Read the model definition and answer for the solid it produces. Units are mm, in the model's axes. Face numbers are marked on the shaded views. Coordinates: 2 decimals unless noted, no trailing zeros. Order: outer loops, then holes, each group sorted by start corner. A loop starts at its lowest first (then second) coordinate and runs counter-clockwise, first axis right, second up. Notation, with made-up numbers: M 82,-38.5 L 100,-38.5 A29 ccw 100,-3.5 Z; hole C -16,-15.75 d11. An arc over 180 degrees is marked long. One line per question, with ' | ' between items. Start each with the question number.
1) The mould has two halves that part along X. Classify the marked faces 1, 2, 3 and 4: +X half, -X half, draft (parallel to the pull), parting line (faces both ways), or undercut.
2) Find section C-C, the plane z = 15.5. Write down the section's boundary in (x, y), plus the area to 3 significant figures.
3) Find section A-A, the plane x = 10.6. Write down the section's boundary in (y, z).
4) Given P1, Ø3, axis at x = -1, z = 12, coming from the -Y side; P2, Ø1.5, axis at y = 19, z = 2, coming from the -X side; P3, Ø2, axis at x = 24.5, y = -23.5, coming from the +Z side, each flat-ended and moving along its own axis, determine where each tip first touches the part or whether it passes through.
5) Find section D-D, the plane x = 0. Write down the section's boundary in (y, z), plus the area to 3 significant figures.
6) Consider probe 1 along Y at (x, z) = (0, 10.25); probe 2 along Y at (x, z) = (0, 1.5); probe 3 along Z at (x, y) = (14, -30). Determine where each line is inside the solid, lowest interval first.
7) Find section B-B, the plane y = -16. Write down the section's boundary in (x, z), plus the area to 3 significant figures.
from build123d import *

# Parameters (mm, degrees)
ESQUISSE1_R             = 35
BOSS_EXTRU_1_DEPTH      = 5
ENL_V_MAT_EXTRU_1_REACH = 51.749
BOSS_EXTRU_3_OUTLINE_R  = 4.75
BOSS_EXTRU_3_DEPTH      = 12


# Read off the part's stored shape, not the designer's step: Boss.-Extru.3
with BuildPart() as part:
    # Esquisse1 → Boss.-Extru.1 (new body)
    with BuildSketch(Plane.XY):
        Circle(ESQUISSE1_R)
        with BuildLine():
            ThreePointArc((4.728110875, -10.282810642), (4.727635283, -10.351772147), (4.726208599, -10.420720532))
            Line((4.726208599, -10.420720532), (4.312478928, -25.415013705))
            ThreePointArc((4.312478928, -25.415013705), (-0.823528687, -30.275201539), (-5.683716521, -25.139193925))
            Line((-5.683716521, -25.139193925), (-5.26998685, -10.144900751))
            ThreePointArc((-5.26998685, -10.144900751), (-0.202927621, -5.283286233), (4.728110875, -10.282810642))
        make_face(mode=Mode.SUBTRACT)
        with BuildLine():
            Line((-8.268845484, -10.062154817), (-8.682575156, -25.05644799))
            ThreePointArc((-8.682575156, -25.05644799), (-11.353299115, -27.583745664), (-13.880596789, -24.913021704))
            Line((-13.880596789, -24.913021704), (-13.466867118, -9.918728531))
            ThreePointArc((-13.466867118, -9.918728531), (-10.796143158, -7.391430858), (-8.268845484, -10.062154817))
        make_face(mode=Mode.SUBTRACT)
        with BuildLine():
            Line((12.923088867, -10.646892753), (12.509359196, -25.641185926))
            ThreePointArc((12.509359196, -25.641185926), (9.838635236, -28.168483599), (7.311337562, -25.49775964))
            Line((7.311337562, -25.49775964), (7.725067233, -10.503466467))
            ThreePointArc((7.725067233, -10.503466467), (10.395791193, -7.976168793), (12.923088867, -10.646892753))
        make_face(mode=Mode.SUBTRACT)
        with BuildLine():
            Line((-13.2, 10), (-13.2, 25))
            ThreePointArc((-13.2, 25), (-10.6, 27.6), (-8, 25))
            Line((-8, 25), (-8, 10))
            ThreePointArc((-8, 10), (-10.6, 7.4), (-13.2, 10))
        make_face(mode=Mode.SUBTRACT)
        with BuildLine():
            ThreePointArc((5, 10), (0, 5), (-5, 10))
            Line((-5, 10), (-5, 25))
            ThreePointArc((-5, 25), (0, 30), (5, 25))
            Line((5, 25), (5, 10))
        make_face(mode=Mode.SUBTRACT)
        with BuildLine():
            ThreePointArc((8, 25), (10.6, 27.6), (13.2, 25))
            Line((13.2, 25), (13.2, 10))
            ThreePointArc((13.2, 10), (10.6, 7.4), (8, 10))
            Line((8, 10), (8, 25))
        make_face(mode=Mode.SUBTRACT)
    extrude(amount=BOSS_EXTRU_1_DEPTH)

    # Esquisse2 → Enl_v. mat.-Extru.1 (cut, up to next)
    with BuildSketch(Plane.XY.offset(5), mode=Mode.PRIVATE) as enl_v_mat_extru_1_sk1:
        with BuildLine():
            Line((1.833030278, 2.05), (-1.833030278, 2.05))
            ThreePointArc((-1.833030278, 2.05), (-1.122868366, -2.510312059), (2.75, 0))
            ThreePointArc((2.75, 0), (2.510312059, 1.122868366), (1.833030278, 2.05))
        make_face()
    enl_v_mat_extru_1_tool1 = extrude(enl_v_mat_extru_1_sk1.sketch, amount=-ENL_V_MAT_EXTRU_1_REACH, mode=Mode.PRIVATE) & part.part
    add(enl_v_mat_extru_1_tool1.solids().sort_by_distance((0, -0.186648, 5))[0], mode=Mode.SUBTRACT)

    # Boss.-Extru.3 outline → Boss.-Extru.3 (add)
    with BuildSketch(Plane.XY.offset(5)):
        Circle(BOSS_EXTRU_3_OUTLINE_R)
        with BuildLine():
            ThreePointArc((1.833030278, 2.05), (0, -2.75), (-1.833030278, 2.05))
            Line((-1.833030278, 2.05), (1.833030278, 2.05))
        make_face(mode=Mode.SUBTRACT)
    extrude(amount=BOSS_EXTRU_3_DEPTH)


solid = part.part
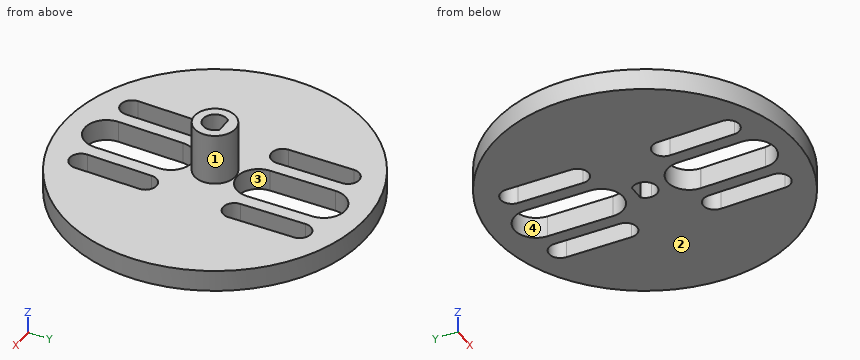
Report:
1) face 1: parting line | face 2: draft | face 3: undercut | face 4: undercut
2) outline: C 0,0 d9.5; hole M -1.83,2.05 A2.75 ccw long 1.83,2.05 Z | area: 48.9 mm^2
3) outline: M -33.36,0 L -28.08,0 L -28.08,5 L -33.36,5 Z; M -7.99,0 L 7.4,0 L 7.4,5 L -7.99,5 Z; M 27.6,0 L 33.36,0 L 33.36,5 L 27.6,5 Z
4) P1: stops at y = -4.75 | P2: stops at x = -29.87 | P3: stops at z = 5
5) outline: M -35,0 L -30.23,0 L -30.23,5 L -35,5 Z; M -5.29,0 L -2.75,0 L -2.75,17 L -4.75,17 L -4.75,5 L -5.29,5 Z; M 2.05,0 L 5,0 L 5,5 L 4.75,5 L 4.75,17 L 2.05,17 Z; M 30,0 L 35,0 L 35,5 L 30,5 Z | area: 133 mm^2
6) probe 1: y = -4.75 to -2.75, 2.05 to 4.75 | probe 2: y = -35 to -30.23, -5.29 to -2.75, 2.05 to 5, 30 to 35 | probe 3: z = 0 to 5
7) outline: M -31.13,0 L -13.63,0 L -13.63,5 L -31.13,5 Z; M -8.43,0 L -5.43,0 L -5.43,5 L -8.43,5 Z; M 4.57,0 L 7.57,0 L 7.57,5 L 4.57,5 Z; M 12.78,0 L 31.13,0 L 31.13,5 L 12.78,5 Z | area: 209 mm^2
